from build123d import *

# Parameters (mm, degrees)
BOSS_EXTRUDE1_DEPTH = 45
SKETCH2_R           = 4
CUT_EXTRUDE1_DEPTH  = 81.932070281
SKETCH3_R           = 2.5
CUT_EXTRUDE3_DEPTH  = 84.815273071


with BuildPart() as part:
    # Sketch1 → Boss-Extrude1 (new body)
    with BuildSketch(Plane.XY):
        Polygon((0, 0), (0, 50), (-5, 50), (-5, 5), (-50, 5), (-50, 0), align=None)
    extrude(amount=BOSS_EXTRUDE1_DEPTH)

    # Sketch2 → Cut-Extrude1 (cut, through all)
    with BuildSketch(Plane.ZY.offset(5)):
        with Locations((15, 40)):
            Circle(SKETCH2_R)
        with Locations((30, 40)):
            Circle(SKETCH2_R)
    extrude(amount=-CUT_EXTRUDE1_DEPTH, mode=Mode.SUBTRACT)

    # Sketch3 → Cut-Extrude3 (cut, through all)
    with BuildSketch(Plane(origin=(0, 0, 0), x_dir=(1, 0, 0), z_dir=(0, 1, 0))):
        with Locations((-35, -30)):
            Circle(SKETCH3_R)
        with Locations((-20, -15)):
            Circle(SKETCH3_R)
    extrude(amount=CUT_EXTRUDE3_DEPTH, mode=Mode.SUBTRACT)


solid = part.part
Input: part model. Units: mm. Frame: model coordinates. A direction names the side the tool comes from. Coordinates: 2 decimals unless noted, no trailing zeros. Loops run counter-clockwise (first coordinate to the right, second up) from the corner with the lowest first, then second, coordinate; pieces in that order, holes last. Notation, with made-up numbers: (-34, -4.75) - (12, -4.75) arc R11 cw to (12, 3.25) - close; hole circle Ø6 at (20.5, -36.75). An arc over 180 degrees is marked (long way). Answer in a Markdown table with one row per item. Add a question column.
Item 1: Section query C-C on z = 15. Return the cut outline in (x, y).
Item 2: Section query B-B on x = -35. Return the cut outline in (y, z).
Item 3: Section query D-D on z = 4.5. Return the cut outline in (x, y).
Item 4: Section query A-A on y = 40. Return the cut outline in (x, z), then the cut area to 3 significant figures.
Item 5: Access query for faces 1 (the cylindrical face through (-33.66, 2.46, 27.89)), 2 (the flat face through (-27, 5, 22)). Directions: +Z, -Z, +X, -X, +Y, -Y. A direction counts if a zero-diameter tool reaches every point of the face in a straight line with its end or side. Return the directions, or none.
Item 6: Line query: line 1 along X through (y, z) = (1.6, 15); line 2 along Y through (x, z) = (-2.95, 15); line 3 along X through (y, z) = (27, 29.5). Output: solid intervals per line, ascending. Write a range as [from, to].
Item 7: Contact query for flat-ended pins moving along their axis: P1, Ø3, axis at y = 15.5, z = 10.5, coming from the -X side; P2, Ø6, axis at x = -35, z = 30, coming from the +Y side. Output: stop coordinate, or through.
Item 8: Mould query, pull axis Z, two halves, no side actions, for faces 3 (the flat face through (-14, 4.7, 45)), 4 (the flat face through (-25, 0, 22)), 5 (the cylindrical face through (-22.5, 2.5, 14.9)). Classes: released by +Z, released by -Z, zero draft, split by the parting line, or undercut.
Recorded:
| question | item | result |
|---|---|---|
| 1 | outline | (-50, 0) - (-22.5, 0) - (-22.5, 5) - (-50, 5) - close; (-17.5, 0) - (0, 0) - (0, 36) - (-5, 36) - (-5, 5) - (-17.5, 5) - close; (-5, 44) - (0, 44) - (0, 50) - (-5, 50) - close |
| 2 | outline | (0, 0) - (5, 0) - (5, 27.5) - (0, 27.5) - close; (0, 32.5) - (5, 32.5) - (5, 45) - (0, 45) - close |
| 3 | outline | (-50, 0) - (0, 0) - (0, 50) - (-5, 50) - (-5, 5) - (-50, 5) - close |
| 4 | outline | (-5, 0) - (0, 0) - (0, 11) - (-5, 11) - close; (-5, 19) - (0, 19) - (0, 26) - (-5, 26) - close; (-5, 34) - (0, 34) - (0, 45) - (-5, 45) - close |
| 4 | area | 145 mm^2 |
| 5 | face 1 | +Y, -Y |
| 5 | face 2 | +Z, -Z, -X, +Y |
| 6 | line 1 | [-50, -22.5], [-17.5, 0] |
| 6 | line 2 | [0, 36], [44, 50] |
| 6 | line 3 | [-5, 0] |
| 7 | P1 | x = -5 |
| 7 | P2 | y = 5 |
| 8 | face 3 | released by +Z |
| 8 | face 4 | zero draft |
| 8 | face 5 | undercut |
